from build123d import *

# Parameters (mm, degrees)
SKETCH043_R     = 2.3
PAD030_DEPTH    = 3
PAD031_DEPTH    = 1.5
POCKET006_DEPTH = 0.6
CHAMFER_SIZE    = 0.1


with BuildPart() as part:
    # Sketch043 → Pad030 (new body)
    with BuildSketch(Plane.XY):
        Circle(SKETCH043_R)
    extrude(amount=PAD030_DEPTH)

    # Sketch044 (on Face3 of Pad030) → Pad031 (join)
    with BuildSketch(Plane.XY.offset(3)):
        with BuildLine():
            Line((0.425, 2.767558), (0.425, 3.617558))
            Line((0.425, 3.617558), (-0.425, 3.617558))
            Line((-0.425, 3.617558), (-0.425, 2.767558))
            ThreePointArc((-0.425, 2.767558), (0, -2.8), (0.425, 2.767558))
        make_face()
    extrude(amount=PAD031_DEPTH)

    # Sketch045 → Pocket006 (cut)
    with BuildSketch(Plane.XY):
        Polygon((-1.443376, -0.9), (0, 1.6), (1.443376, -0.9), align=None)
    extrude(amount=POCKET006_DEPTH, mode=Mode.SUBTRACT)

    # Chamfer
    chamfer_edges = [part.edges().sort_by_distance(p)[0] for p in [
        (-0.721688, 0.35, 0),
        (0, -0.9, 0),
        (0.721688, 0.35, 0),
        (-2.3, 0, 0),
    ]]
    chamfer(chamfer_edges, length=CHAMFER_SIZE)


with BuildPart() as part_1:
    # Body012 placement: moved
    add(part.part.moved(Location((63.6, 11.5, -1.5))))


solid = part_1.part
Part model, mm, in its own coordinate system. A direction names the side the tool comes from. Coordinates: 2 decimals unless noted, no trailing zeros. Loops run counter-clockwise (first coordinate to the right, second up) from the corner with the lowest first, then second, coordinate; pieces in that order, holes last. Notation, with made-up numbers: M -33,52.5 L -14,52.5 A19 ccw -14,80.5 Z; hole C 11,10.5 d8. An arc over 180 degrees is marked long. Use a Markdown table: item, result. Add a question column.
Q1. Probe L1, parallel to X at y = 10.75, z = -1.05; L2, parallel to Z at x = 63.75, y = 11.5; L3, parallel to Z at x = 61.4, y = 10. List the from-to ranges inside material, lowest first.
Q2. Cut at B-B (y = 11.5). Write the cut outline in (x, z).
Q3. Pin check, flat tips, straight feed: P1, Ø0.9, axis at y = 14.5, z = 2.5, coming from the -X side; P2, Ø1.5, axis at x = 62.5, z = 0.5, coming from the +Y side; P3, Ø0.7, axis at y = 15, z = 2.5, coming from the +X side (3 decimals). Stop position of each tip, or through.
Q4. Mould opens along Y. For faces 1 (the flat face through (65, 12, -1.5)), 2 (the flat face through (64, 12, -0.9)), 3 (the cylindrical face through (65.794, 12.191, 0.03)) say: +Y half, -Y half, draft (parallel to the pull), parting line (faces both ways), or undercut.
Q5. Which spindle directions (+Z, -Z, +X, -X, +Y, -Y) get a long thin tool onto all of the face, cutting with end or side? Do faces 4 (the flat face through (64.025, 14.7, 2.2)), 5 (the flat face through (63.175, 14.7, 2.2)), 6 (the flat face through (63.6, 15.118, 2.2)), 7 (the flat face through (64, 14, 1.5)). Say none if no direction does.
Q6. Cut at C-C (z = 2.75). Write the cut outline in (x, y) (3 decimals).
Q7. Cut at D-D (z = 1.4). Write the cut outline in (x, y), and give its area (3 significant figures).
Q8. Cut at A-A (z = -1.1). Write the cut outline in (x, y).
Worked out:
| question | item | result |
|---|---|---|
| 1 | L1 | x = 61.43 to 62.24, 64.96 to 65.77 |
| 1 | L2 | z = -0.9 to 3 |
| 1 | L3 | z = 1.5 to 3 |
| 2 | outline | M 60.8,1.5 L 61.3,1.5 L 61.3,-1.4 L 61.4,-1.5 L 62.56,-1.5 L 62.68,-1.4 L 62.68,-0.9 L 64.52,-0.9 L 64.52,-1.4 L 64.64,-1.5 L 65.8,-1.5 L 65.9,-1.4 L 65.9,1.5 L 66.4,1.5 L 66.4,3 L 60.8,3 Z |
| 3 | P1 | stops at x = 62.44 |
| 3 | P2 | stops at y = 13.77 |
| 3 | P3 | stops at x = 64.025 |
| 4 | face 1 | draft |
| 4 | face 2 | undercut |
| 4 | face 3 | parting line |
| 5 | face 4 | +Z, -Z, +X, +Y |
| 5 | face 5 | +Z, -Z, -X, +Y |
| 5 | face 6 | +Z, -Z, +X, -X, +Y |
| 5 | face 7 | -Z |
| 6 | outline | M 63.175,14.268 A2.8 ccw long 64.025,14.268 L 64.025,15.118 L 63.175,15.118 Z |
| 7 | outline | C 63.6,11.5 d4.6 |
| 7 | area | 16.6 mm2 |
| 8 | outline | C 63.6,11.5 d4.6; hole M 62.16,10.6 L 65.04,10.6 L 63.6,13.1 Z |
